Autodesk Inventor part; units mm, degrees
ref_plane "YZ Plane" through (0, 0, 0) normal (1, 0, 0) x (0, 1, 0)
ref_plane "XZ Plane" through (0, 0, 0) normal (0, 1, 0) x (-1, 0, 0)
ref_plane "XY Plane" through (0, 0, 0) normal (0, 0, 1) x (1, 0, 0)
sketch "Sketch1" plane through (0, 0, 0) normal (0, 1, 0) x (-1, 0, 0)
  circle A0 centre (0, 0) radius 6.1
  dimension "d0" = 12.2
extrude "Extrusion1" add sketch "Sketch1" along normal blind 3.5
sketch "Sketch2" plane through (0, 3.5, 0) normal (0, 1, 0) x (1, 0, 0)
  circle A0 centre (0, 0) radius 1.5
  dimension "d3" = 3
extrude "Extrusion2" cut sketch "Sketch2" against normal blind 1
sketch "Sketch3" plane through (0, 0, 0) normal (0, -1, 0) x (1, 0, 0)
  circle A0 centre (0, 0) radius 5
  circle A1 centre (0, 0) radius 6.1
  dimension "d6" = 10
extrude "Extrusion3" cut sketch "Sketch3" against normal blind 0.5
sketch "Sketch4" plane through (0, 0, 0) normal (0, 1, 0) x (-1, 0, 0)
  line L0 (-8.54, 0) -> (8.54, 0) construction
  circle A0 centre (-2.5, 0) radius 0.325
  circle A1 centre (2.5, 0) radius 0.325
  line L1 (0, -8.54) -> (0, 8.54) construction
  point P0 (0, 0)
  dimension "d9" = 0.65
  dimension "d10" = 0.65
  dimension "d11" = 5
extrude "Extrusion4" add sketch "Sketch4" against normal blind 3
sketch "Sketch5" plane through (0, 0, 0) normal (0, -1, 0) x (1, 0, 0)
  line L0 (0, 8.54) -> (0, -8.54) construction
  line L1 (-8.54, 0) -> (8.54, 0) construction
  circle A0 centre (0, -4.5) radius 0.25
  circle A1 centre (0, 4.5) radius 0.25
  point P0 (0, 0)
  dimension "d14" = 0.5
  dimension "d15" = 0.5
  dimension "d16" = 9
extrude "Extrusion5" add sketch "Sketch5" along normal blind 0.6
properties part number "BUZZER_TDK_PS12"
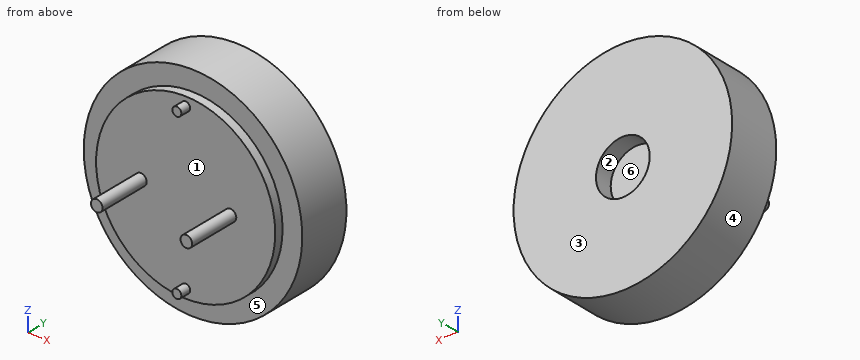
CAD build for the part. Positions are in the model's coordinates, mm. Face numbers are marked on the shaded views. A direction names the side the tool comes from. Round coordinates to 2 decimals unless told otherwise and drop trailing zeros. Write each loop counter-clockwise with the first axis right and the second up, starting at its lowest first coordinate (ties: lowest second). Pieces come first, ordered by that corner, then holes. Notation, with made-up numbers: M -28.75,-11 L 8.25,-11 A32 ccw 8.25,27 Z; hole C -35,21.25 d5. An arc over 180 degrees is marked long. Put each result on its own line as item: value. Start each with the question number.
1) Drill centre lines: probe 1 along Z at (x, y) = (0, 3.2); probe 2 along Y at (x, z) = (2.5, -1); probe 3 along Y at (x, z) = (0.5, -1). Where is each one in solid material? Low to high. Write a range as [from, to].
2) Pull direction X, two halves, no side cores. Call the marked faces 4, 5 and 6: pulls with the +X half, pulls with the -X half, needs draft (parallel to the pull), parting line crosses it, or undercut.
3) Saw through at B-B, the plane x = 0. Write the cut outline in (y, z), and give its area (3 significant figures).
4) Saw through at D-D, the plane y = 1. Write the cut outline in (x, z), and give its area (3 significant figures).
5) Saw through at C-C, the plane y = -2. Write the cut outline in (x, z) (3 decimals), and give its area (3 significant figures).
6) 3-axis set-ups, long thin cutter, end or side, ignore diameter. For the marked faces 1, 2 and 3: which of +Z, -Z, +X, -X, +Y, -Y reach the whole face in a straight line?
7) Pin check, flat tip, straight feed: pin 1 Ø1.5 at (x, z) = (-0.5, 0) entering from +Y. Stop position of the tip, or through.
8) Saw through at A-A, the plane z = 0. Write the cut outline in (x, y) (3 decimals).
Resolved:
1. probe 1: [-6.1, -1.5], [1.5, 6.1]
1. probe 2: [0, 3.5]
1. probe 3: [0, 2.5]
2. face 4: parting line crosses it
2. face 5: needs draft
2. face 6: undercut
3. outline: M -0.6,-4.75 L 0,-4.75 L 0,-5 L 0.5,-5 L 0.5,-6.1 L 3.5,-6.1 L 3.5,-1.5 L 2.5,-1.5 L 2.5,1.5 L 3.5,1.5 L 3.5,6.1 L 0.5,6.1 L 0.5,5 L 0,5 L 0,4.75 L -0.6,4.75 L -0.6,4.25 L 0,4.25 L 0,-4.25 L -0.6,-4.25 Z
3. area: 39.2 mm²
4. outline: C 0,0 d12.2
4. area: 117 mm²
5. outline: C -2.5,0 d0.65; C 2.5,0 d0.65
5. area: 0.664 mm²
6. face 1: -Y
6. face 2: +Y
6. face 3: +Z, -Z, +X, -X, +Y
7. pin 1: y = 2.5
8. outline: M -6.1,0.5 L -5,0.5 L -5,0 L -2.825,0 L -2.825,-3 L -2.175,-3 L -2.175,0 L 2.175,0 L 2.175,-3 L 2.825,-3 L 2.825,0 L 5,0 L 5,0.5 L 6.1,0.5 L 6.1,3.5 L 1.5,3.5 L 1.5,2.5 L -1.5,2.5 L -1.5,3.5 L -6.1,3.5 Z
